```python
from build123d import *

# Parameters (mm, degrees)
SKETCH_1_W          = 35
SKETCH_1_H          = 25
SKETCH_1_R          = 8
EXTRUDE_2_DEPTH     = 25
SKETCH_2_R          = 8
EXTRUDE_3_DEPTH     = 5
EXTRUDE_START       = 10
SKETCH_3_R          = 8
EXTRUDE_4_DEPTH     = 10
SKETCH_4_R          = 3
CUT_EXTRUDE_1_DEPTH = 46.414755311
SKETCH_5_R          = 11.5
CUT_EXTRUDE_2_DEPTH = 16
SKETCH_6_R          = 4
EXTRUDE_5_DEPTH     = 15
SKETCH_8_W          = 3
SKETCH_8_H          = 2.025472792
CUT_EXTRUDE_3_DEPTH = 15
EXTRUDE_START_2     = -2
SKETCH_9_R          = 4
EXTRUDE_6_DEPTH     = 2
SKETCH_10_R         = 4
EXTRUDE_7_DEPTH     = 2
EXTRUDE_START_3     = 3
SKETCH_12_R         = 3
SKETCH_12_R_2       = 8
EXTRUDE_11_DEPTH    = 3
SKETCH_14_W         = 6.627877622
SKETCH_14_H         = 25
CUT_EXTRUDE_4_DEPTH = 3
SKETCH_15_W         = 25
SKETCH_15_H         = 25
CUT_EXTRUDE_5_DEPTH = 70.862501092
SKETCH_16_W         = 25
SKETCH_16_H         = 25
SKETCH_16_R         = 4
EXTRUDE_12_DEPTH    = 1


with BuildPart() as part:
    # 草图1 → 凸台-拉伸2 (new body)
    # profile 1 of 2: a face of its own
    with BuildSketch(Plane.XY):
        Rectangle(SKETCH_1_W, SKETCH_1_H)
        with Locations((9.5, 0)):
            Circle(SKETCH_1_R, mode=Mode.SUBTRACT)
    # profile 2 of 2: a face of its own
    with BuildSketch(Plane.XY):
        with Locations((9.5, 0)):
            Circle(SKETCH_1_R)
    extrude(amount=EXTRUDE_2_DEPTH)

    # 草图2 → 凸台-拉伸3 (add)
    with BuildSketch(Plane.XY.offset(25)):
        with Locations((9.5, 0)):
            Circle(SKETCH_2_R)
    extrude(amount=EXTRUDE_3_DEPTH)

    # 草图3 → 凸台-拉伸4 (add)
    with BuildSketch(Plane(origin=(0, 0, 0), x_dir=(-1, 0, 0), z_dir=(0, 0, -1)).offset(EXTRUDE_START)):
        with Locations(Location((-9.5, 0, 0), (0, 0, 180))):
            Circle(SKETCH_3_R)
    extrude(amount=-EXTRUDE_4_DEPTH)

    # 草图4 → 切除-拉伸1 (cut, through all)
    with BuildSketch(Plane.XY.offset(30)):
        with Locations((9.5, 0)):
            Circle(SKETCH_4_R)
    extrude(amount=-CUT_EXTRUDE_1_DEPTH, mode=Mode.SUBTRACT)

    # 草图5 → 切除-拉伸2 (cut)
    with BuildSketch(Plane(origin=(17.5, 0, 0), x_dir=(0, 0, -1), z_dir=(1, 0, 0))):
        with Locations((-12.5, 0)):
            Circle(SKETCH_5_R)
    extrude(amount=-CUT_EXTRUDE_2_DEPTH, mode=Mode.SUBTRACT)

    # 草图6 → 凸台-拉伸5 (add)
    with BuildSketch(Plane.ZY.offset(17.5)):
        with Locations((12.5, 0)):
            Circle(SKETCH_6_R)
    extrude(amount=EXTRUDE_5_DEPTH)

    # 草图8 → 切除-拉伸3 (cut)
    with BuildSketch(Plane.ZY.offset(17.5)):
        with Locations((17, 0)):
            Rectangle(SKETCH_8_W, SKETCH_8_H)
    extrude(amount=CUT_EXTRUDE_3_DEPTH, mode=Mode.SUBTRACT)

    # 草图9 → 凸台-拉伸6 (add)
    with BuildSketch(Plane.ZY.offset(32.5).offset(EXTRUDE_START_2)):
        with Locations(Location((12.5, 0, 0), (0, 0, 14.666011097))):
            Circle(SKETCH_9_R)
    extrude(amount=EXTRUDE_6_DEPTH)

    # 草图10 → 凸台-拉伸7 (add)
    with BuildSketch(Plane.ZY.offset(17.5)):
        with Locations((12.5, 0)):
            Circle(SKETCH_10_R)
    extrude(amount=EXTRUDE_7_DEPTH)

    # 草图12 → 凸台-拉伸11 (add)
    with BuildSketch(Plane(origin=(0, 0, 0), x_dir=(-1, 0, 0), z_dir=(0, 0, -1)).offset(EXTRUDE_START_3)):
        Polygon((12.5, 12.5), (-24.127877622, 12.5), (-24.127877622, -12.5), (-17.5, -12.5), (-32.5, -38.480762114), (12.5, -12.5), align=None)
        with Locations((-17.5, -25.490381057)):
            Circle(SKETCH_12_R, mode=Mode.SUBTRACT)
        with Locations(Location((-9.5, 0, 0), (0, 0, 180))):
            Circle(SKETCH_12_R_2, mode=Mode.SUBTRACT)
    extrude(amount=-EXTRUDE_11_DEPTH)

    # 草图14 → 切除-拉伸4 (cut)
    with BuildSketch(Plane.XY):
        with Locations((20.813938811, 0)):
            Rectangle(SKETCH_14_W, SKETCH_14_H)
    extrude(amount=-CUT_EXTRUDE_4_DEPTH, mode=Mode.SUBTRACT)

    # 草图15 → 切除-拉伸5 (cut, through all)
    with BuildSketch(Plane.ZY.offset(17.5)):
        with Locations((12.5, 0)):
            Rectangle(SKETCH_15_W, SKETCH_15_H)
    extrude(amount=CUT_EXTRUDE_5_DEPTH, mode=Mode.SUBTRACT)

    # 草图16 → 凸台-拉伸12 (add)
    with BuildSketch(Plane.ZY.offset(17.5)):
        with Locations((12.5, 0)):
            Rectangle(SKETCH_16_W, SKETCH_16_H)
        with Locations((12.5, 0)):
            Circle(SKETCH_16_R, mode=Mode.SUBTRACT)
    extrude(amount=EXTRUDE_12_DEPTH)


solid = part.part
```
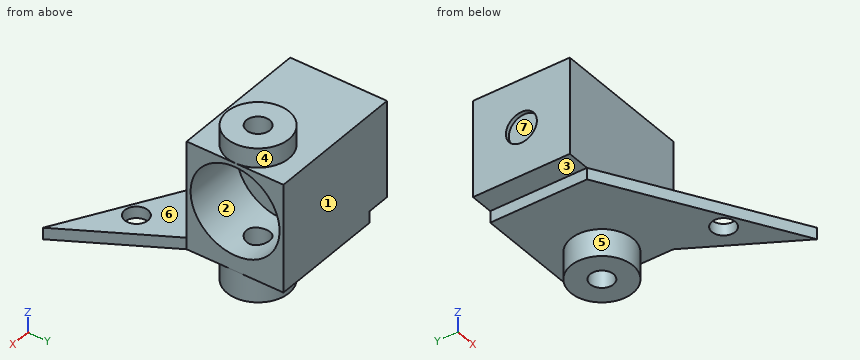
Can you work these out from the model? Positions are in its coordinate system, mm. Face numbers are marked on the shaded views. A direction names the side the tool comes from. Give positions to 0.01 mm unless a question says otherwise; leave off trailing zeros. Write each loop counter-clockwise with the first axis right and the second up, starting at its lowest first coordinate (ties: lowest second). Pieces come first, ordered by that corner, then holes. Notation, with made-up numbers: (27, 27) - (60, 27) arc R22 ccw to (60, 57) - close; hole circle Ø7 at (44, 10.5). An arc over 180 degrees is marked (long way). Write item = value, one per line. Start each with the question number.
1. On a 3-axis mill with a long thin cutter (end or side, diameter ignored), from which of +Z, -Z, +X, -X, +Y, -Y can I reach the whole of each face in a straight line? I mean the marked faces 4, 5, 6 and 7. Say none if no direction works.
2. For pin 1 (20 mm diameter, centred on x = 0.5, z = 16, fed in from -Y); pin 2 (3 mm diameter, centred on x = 22.5, y = -29.5, fed in from +Z); pin 3 (3.5 mm diameter, centred on y = 4, z = -1.5, fed in from -X); pin 4 (6.5 mm diameter, centred on x = -15.5, y = -1, fed in from -Z), each with a flat end and sliding along its axis, tell me the tip position at first contact or that it passes through.
3. Please list where these lines run through material, in increasing order: line 1 (Y direction, x = 9.5, z = -5.25); line 2 (Y direction, x = 14.5, z = 12.5); line 3 (Y direction, x = -17, z = 12).
4. Imagine slicing it at D-D (z = -5). Please give me the cut outline in (x, y).
5. Imagine slicing it at B-B (x = 5.5). Please give me the cut outline in (y, z), and give its area (3 significant figures).
6. Imagine slicing it at A-A (z = 12.5). Please give me the cut outline in (x, y).
7. Imagine slicing it at C-C (y = -26.5). Please give me the cut outline in (x, z) (3 decimals), and give its area (3 significant figures).
8. Thinking about a two-plate mould opening in Y: for the marked faces 1, 2 and 3, which applies, released by +Y, released by -Y, zero draft, split by the parting line, or undercut?
Worked answers:
q1.face_4 = +Z
q1.face_5 = -Z
q1.face_6 = +Z, +X, -X, -Y
q1.face_7 = -X
q2.pin_1 = -12.5
q2.pin_2 = 0
q2.pin_3 = -18.5
q2.pin_4 = -3
q3.line_1 = -8 to -3, 3 to 8
q3.line_2 = -12.5 to -11.5, 11.5 to 12.5
q3.line_3 = -12.5 to 12.5
q4.outline = circle Ø16 at (9.5, 0); hole circle Ø6 at (9.5, 0)
q5.outline = (-22.89, -3) - (-6.93, -3) - (-6.93, -10) - (6.93, -10) - (6.93, -3) - (12.5, -3) - (12.5, 25) - (6.93, 25) - (6.93, 30) - (-6.93, 30) - (-6.93, 25) - (-12.5, 25) - (-12.5, 0) - (-22.89, 0) - close; hole circle Ø23 at (0, 12.5)
q5.area = 482 mm2
q6.outline = (-18.5, -12.5) - (17.5, -12.5) - (17.5, -11.5) - (1.5, -11.5) - (1.5, 11.5) - (17.5, 11.5) - (17.5, 12.5) - (-18.5, 12.5) - (-18.5, 4) - (-17.5, 4) - (-17.5, -4) - (-18.5, -4) - close
q7.outline = (11.749, -3) - (14.675, -3) - (14.675, 0) - (11.749, 0) - close; (20.325, -3) - (25.583, -3) - (25.583, 0) - (20.325, 0) - close
q7.area = 24.6 mm2
q8.face_1 = released by +Y
q8.face_2 = undercut
q8.face_3 = zero draft
